Design review of the part built by this model. Coordinates are the model's own, in mm. Give positions to 0.01 mm unless a question says otherwise; leave off trailing zeros. Answer as a JSON object with one key per item and string values.
```python
from build123d import *


with BuildPart() as f1:
    # F0 (on Front) → F1 (revolve)
    with BuildSketch(Plane.XZ):
        with BuildLine():
            Line((0, 8.8382818858), (0, 0))
            Line((0, 0), (10, 0))
            Line((10, 0), (10, 2))
            Line((10, 2), (9, 2))
            ThreePointArc((9, 2), (9.2928932188, 2.7071067812), (10, 3))
            add(Edge.make_bspline(
                [(10, 3), (5.6970222105, 5.5161274686), (-1.3836503017, 24.4209409655), (6.6211349569, 35.1973583272), (1.3998154741, 39.0954037275)],
                knots=[0, 0, 0, 0, 0.5419605204, 0.9666014846, 0.9666014846, 0.9666014846, 0.9666014846], degree=3))
            ThreePointArc((1.3998154741, 39.0954037275), (0.7969056794, 38.5361970365), (0, 38.3333333333))
            Line((0, 38.3333333333), (0, 37.6222543418))
            Line((0, 37.6222543418), (2.2149570286, 35.4595184326))
            Line((2.2149570286, 35.4595184326), (2.2149570286, 32.5758717954))
            Line((2.2149570286, 32.5758717954), (1.3498631306, 27.0969439298))
            Line((1.3498631306, 27.0969439298), (0.9173162398, 21.1133789271))
            Line((0.9173162398, 21.1133789271), (1.9265923183, 13.3996251971))
            Line((1.9265923183, 13.3996251971), (3.0079598073, 9.722976014))
            Line((3.0079598073, 9.722976014), (0, 8.8382818858))
        make_face()
        with BuildLine():
            Line((0, 41.6666666667), (0, 40))
            add(Edge.make_bspline(
                [(1.3998154741, 39.0954037275), (0.9891525046, 39.4019896211), (0.5244366288, 39.7034029043), (0, 40)],
                knots=[0.9666014846, 0.9666014846, 0.9666014846, 0.9666014846, 1, 1, 1, 1], degree=3))
            ThreePointArc((1.3998154741, 39.0954037275), (1.4638029635, 40.7969056794), (0, 41.6666666667))
        make_face()
        with BuildLine():
            Line((0, 40), (0, 38.3333333333))
            ThreePointArc((0, 38.3333333333), (0.7969056794, 38.5361970365), (1.3998154741, 39.0954037275))
            add(Edge.make_bspline(
                [(1.3998154741, 39.0954037275), (0.9891525046, 39.4019896211), (0.5244366288, 39.7034029043), (0, 40)],
                knots=[0.9666014846, 0.9666014846, 0.9666014846, 0.9666014846, 1, 1, 1, 1], degree=3))
        make_face()
    revolve(axis=Axis((0, 0, 20), (0, 0, 1)))


solid = f1.part
```
(1) Clearance check with flat-ended pins moving along their axes: pin 1 (5 mm diameter, centred on y = -3.5, z = 13, fed in from -X); pin 2 (6 mm diameter, centred on x = 7.5, z = 19, fed in from +Y); pin 3 (4 mm diameter, centred on x = -3.5, z = 17, fed in from +Y); pin 4 (2 mm diameter, centred on x = -0.5, z = 30, fed in from -Y). State where each tip first meets the part, or that it passes through.
Here are the results:
{"pin 1": "stops at x = -4.1", "pin 2": "passes through", "pin 3": "stops at y = 2.53", "pin 4": "stops at y = -3.86"}
(2) The part is to be moulded in two halves that separate along Y. For faces 1 (the cylindrical face through (-2.17, -9.76, 1.01)), 2 (the conical face through (-0.15, 1.12, 24.06)), 3 (the flat face through (0, 0, 0)), say which applies: +Y half, -Y half, draft (parallel to the pull), parting line (faces both ways), or undercut.
Here are the results:
{"face 1": "parting line", "face 2": "undercut", "face 3": "draft"}
(3) For line 1 along Y through (x, z) = (0, 33.55); line 2 along Z through (x, y) = (-4, 4.75); line 3 along X through (y, z) = (0.5, 22.5), list the stretches that pass through material, from the lowest coordinate up.
Here are the results:
{"line 1": "y = -4.21 to -2.21, 2.21 to 4.21", "line 2": "z = 0 to 7.38", "line 3": "x = -2.35 to -0.89, 0.89 to 2.35"}
